Build history of the part. All positions in model axes, mm. A direction names the side the tool comes from. Give positions to 0.01 mm unless a question says otherwise; leave off trailing zeros. Order: outer loops, then holes, each group sorted by start corner. A loop starts at its lowest first (then second) coordinate and runs counter-clockwise, first axis right, second up. Notation, with made-up numbers: (78.5, 63.5) - (124.5, 63.5) arc R21 ccw to (124.5, 91.5) - close; hole circle Ø2 at (33.25, 26.25). An arc over 180 degrees is marked (long way). Use a Markdown table: item, result. Add a question column.
(1) Flat gauge pins, fed straight in: pin 1 (3 mm diameter, centred on x = 3498.5, z = 2.5, fed in from +Y); pin 2 (3 mm diameter, centred on x = 3500, z = 3, fed in from +Y); pin 3 (1.6 mm diameter, centred on x = 3500, z = 2.5, fed in from -Y). Where does each tip first touch, or does it go through?
(2) Slice it at B-B (y = 1388). Write the cut outline in (x, z).
(3) Slice it at C-C (z = 1.2). Count the separate pieces of the cut face and the enclosed holes in it, then the cut area to 3 significant figures.
(4) Which spindle directions (+Z, -Z, +X, -X, +Y, -Y) get a long thin tool onto all of the face, cutting with end or side? Do faces 1 (the face through (3434.843, 1396, 3)), 2 (the face through (3434, 1381.05, 3)), 3 (the face through (3426.343, 1378, 3)), 4 (the face through (3503.093, 1407, 3)). Say none if no direction does.
(5) Slice it at A-A (y = 1401). Write the cut outline in (x, z), then the cut area to 3 significant figures.
(6) Slice it at D-D (y = 1413.5). Write the cut outline in (x, z), then the cut area to 3 significant figures.
(7) Wall check: line 1 (X direction, y = 1403, z = 0.85); line 2 (X direction, y = 1405.5, z = 2.5); line 3 (X direction, y = 1401, z = 0.3). Give the ranges that are in metal, low to high.
from build123d import *

# Parameters (mm, degrees)
MODEL_W             = 5.5
MODEL_H             = 5.5
BOSS_EXTRUDE1_DEPTH = 6


with BuildPart() as part:
    # Model → Boss-Extrude1 (new body)
    with BuildSketch(Plane.XY):
        with BuildLine():
            Line((3413.843002063, 1402.049969321), (3413.843002063, 1381.049969321))
            Line((3413.843002063, 1381.049969321), (3426.343002063, 1381.049969321))
            Line((3426.343002063, 1381.049969321), (3426.343002063, 1375.049969321))
            Line((3426.343002063, 1375.049969321), (3432.343002063, 1375.049969321))
            Line((3432.343002063, 1375.049969321), (3432.343002063, 1381.049969321))
            Line((3432.343002063, 1381.049969321), (3434.843002063, 1381.049969321))
            Line((3434.843002063, 1381.049969321), (3434.843002063, 1412.049969321))
            Line((3434.843002063, 1412.049969321), (3425.081211359, 1412.049969321))
            ThreePointArc((3425.081211359, 1412.049969321), (3464.843002063, 1443.049969321), (3504.604792768, 1412.049969321))
            Line((3504.604792768, 1412.049969321), (3494.843002063, 1412.049969321))
            Line((3494.843002063, 1412.049969321), (3494.843002063, 1381.049969321))
            Line((3494.843002063, 1381.049969321), (3505.843002063, 1381.049969321))
            Line((3505.843002063, 1381.049969321), (3515.843002063, 1381.049969321))
            Line((3515.843002063, 1381.049969321), (3515.843002063, 1402.049969321))
            ThreePointArc((3515.843002063, 1402.049969321), (3464.843002063, 1453.049969321), (3413.843002063, 1402.049969321))
        make_face()
        with Locations((3500.343002063, 1386.549969321)):
            Rectangle(MODEL_W, MODEL_H, mode=Mode.SUBTRACT)
        with Locations((3500.343002063, 1406.549969321)):
            Rectangle(MODEL_W, MODEL_H, mode=Mode.SUBTRACT)
        with Locations((3429.343002063, 1386.549969321)):
            Rectangle(MODEL_W, MODEL_H, mode=Mode.SUBTRACT)
        with Locations((3429.343002063, 1406.549969321)):
            Rectangle(MODEL_W, MODEL_H, mode=Mode.SUBTRACT)
    extrude(amount=BOSS_EXTRUDE1_DEPTH)


solid = part.part
Solution:
| question | item | result |
|---|---|---|
| 1 | pin 1 | y = 1441.63 |
| 1 | pin 2 | y = 1440.37 |
| 1 | pin 3 | y = 1381.05 |
| 2 | outline | (3413.84, 0) - (3426.59, 0) - (3426.59, 6) - (3413.84, 6) - close; (3432.09, 0) - (3434.84, 0) - (3434.84, 6) - (3432.09, 6) - close; (3494.84, 0) - (3497.59, 0) - (3497.59, 6) - (3494.84, 6) - close; (3503.09, 0) - (3515.84, 0) - (3515.84, 6) - (3503.09, 6) - close |
| 3 | separate pieces | 1 |
| 3 | enclosed holes | 4 |
| 3 | area | 2,450 mm2 |
| 4 | face 1 | +Z, -Z, -Y |
| 4 | face 2 | +Z, -Z, +X, -Y |
| 4 | face 3 | +Z, -Z, -X, -Y |
| 4 | face 4 | +Z, -Z |
| 5 | outline | (3413.84, 0) - (3434.84, 0) - (3434.84, 6) - (3413.84, 6) - close; (3494.84, 0) - (3515.84, 0) - (3515.84, 6) - (3494.84, 6) - close |
| 5 | area | 252 mm2 |
| 6 | outline | (3415.14, 0) - (3425.47, 0) - (3425.47, 6) - (3415.14, 6) - close; (3504.21, 0) - (3514.54, 0) - (3514.54, 6) - (3504.21, 6) - close |
| 6 | area | 124 mm2 |
| 7 | line 1 | 3413.85 to 3434.84, 3494.84 to 3515.83 |
| 7 | line 2 | 3413.96 to 3426.59, 3432.09 to 3434.84, 3494.84 to 3497.59, 3503.09 to 3515.73 |
| 7 | line 3 | 3413.84 to 3434.84, 3494.84 to 3515.84 |
